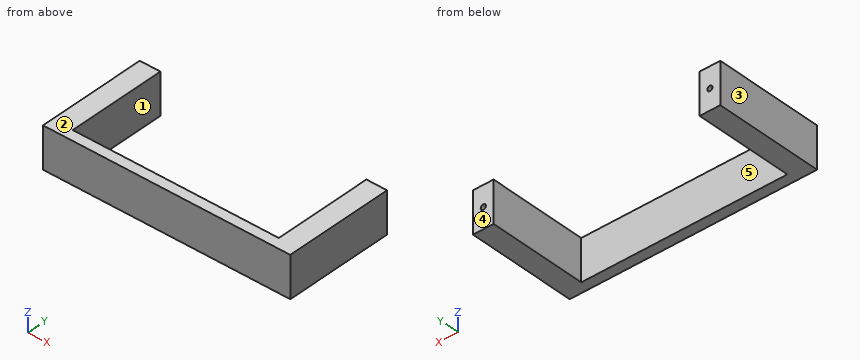
from build123d import *

# Parameters (mm, degrees)
CROQUIS1_W              = 120
CROQUIS1_H              = 20
SALIENTE_EXTRUIR1_DEPTH = 5
CROQUIS2_W              = 10
CROQUIS2_H              = 20
SALIENTE_EXTRUIR2_DEPTH = 48
CROQUIS3_R              = 1.25
CORTAR_EXTRUIR1_DEPTH   = 10


with BuildPart() as part:
    # Croquis1 → Saliente-Extruir1 (new body)
    with BuildSketch(Plane(origin=(0, 0, 0), x_dir=(1, 0, 0), z_dir=(0, 1, 0))):
        Rectangle(CROQUIS1_W, CROQUIS1_H)
    extrude(amount=SALIENTE_EXTRUIR1_DEPTH)

    # Croquis2 → Saliente-Extruir2 (add)
    with BuildSketch(Plane(origin=(0, 5, 0), x_dir=(1, 0, 0), z_dir=(0, 1, 0))):
        with Locations((55, 0)):
            Rectangle(CROQUIS2_W, CROQUIS2_H)
        with Locations((-55, 0)):
            Rectangle(CROQUIS2_W, CROQUIS2_H)
    extrude(amount=SALIENTE_EXTRUIR2_DEPTH)

    # Croquis3 → Cortar-Extruir1 (cut)
    with BuildSketch(Plane(origin=(0, 53, 0), x_dir=(1, 0, 0), z_dir=(0, 1, 0))):
        with Locations(Location((-55, 0, 0), (0, 0, 270))):
            Circle(CROQUIS3_R)
        with Locations(Location((55, 0, 0), (0, 0, 270))):
            Circle(CROQUIS3_R)
    extrude(amount=-CORTAR_EXTRUIR1_DEPTH, mode=Mode.SUBTRACT)


solid = part.part
Verification items for the finished model (mm, model axes). Face numbers are marked on the shaded views. A direction names the side the tool comes from. Give positions to 0.01 mm unless a question says otherwise; leave off trailing zeros. Order: outer loops, then holes, each group sorted by start corner. A loop starts at its lowest first (then second) coordinate and runs counter-clockwise, first axis right, second up. Notation, with made-up numbers: M 20,39 L 45,39 A13 ccw 45,59 Z; hole C 56.25,73 d9. An arc over 180 degrees is marked long. Use one line per item in the form item = value. Start each with the question number.
Q1. Mould release check, pull along X, two halves, no side actions. Record for the marked faces 3, 4 and 5: +X half, -X half, draft (parallel to the pull), parting line (faces both ways), or undercut.
Q2. Go/stop test with flat-tipped pins: pin 1 Ø0.8 at (x, z) = (-55, -0.5) entering from +Y; pin 2 Ø3 at (x, z) = (-28, -5.5) entering from +Y. Record where each tip stops, or that it passes through.
Q3. Section check C-C (z = -8). Enter the section's corners in (x, y).
Q4. Scan lines: line 1 along X through (y, z) = (48.5, 0); line 2 along X through (y, z) = (15, 4.75); line 3 along Y through (x, z) = (9, 3.5). Record each from-to range of solid material in increasing order. Write a range as [from, to].
Q5. Section check A-A (y = 49). Enter the section's corners in (x, z).
Q6. Section check B-B (y = 28.5). Enter the section's corners in (x, z), then the cut area to 3 significant figures.
Q7. Access from +Z, -Z, +X, -X, +Y, -Y to the whole of each face (thin tool, end or side, straight path). Record for the marked faces 1 and 2.
Q8. Section check D-D (x = -55). Enter the section's corners in (y, z), then the cut area to 4 significant figures.
Evaluation:
q1.face_3 = -X half
q1.face_4 = draft
q1.face_5 = undercut
q2.pin_1 = 43
q2.pin_2 = 5
q3.outline = M -60,0 L 60,0 L 60,53 L 50,53 L 50,5 L -50,5 L -50,53 L -60,53 Z
q4.line_1 = [-60, -56.25], [-53.75, -50], [50, 53.75], [56.25, 60]
q4.line_2 = [-60, -50], [50, 60]
q4.line_3 = [0, 5]
q5.outline = M -60,-10 L -50,-10 L -50,10 L -60,10 Z; M 50,-10 L 60,-10 L 60,10 L 50,10 Z; hole C -55,0 d2.5; hole C 55,0 d2.5
q6.outline = M -60,-10 L -50,-10 L -50,10 L -60,10 Z; M 50,-10 L 60,-10 L 60,10 L 50,10 Z
q6.area = 400 mm2
q7.face_1 = +Z, -Z, +Y
q7.face_2 = +Z, +X, -X, +Y, -Y
q8.outline = M 0,-10 L 53,-10 L 53,-1.25 L 43,-1.25 L 43,1.25 L 53,1.25 L 53,10 L 0,10 Z
q8.area = 1,035 mm2
